Autodesk Inventor part; units mm, degrees
ref_plane "YZ Plane" through (0, 0, 0) normal (1, 0, 0) x (0, 1, 0)
ref_plane "XZ Plane" through (0, 0, 0) normal (0, 1, 0) x (-1, 0, 0)
ref_plane "XY Plane" through (0, 0, 0) normal (0, 0, 1) x (1, 0, 0)
sketch "Sketch1" plane through (0, 0, 0) normal (0, 0, 1) x (1, 0, 0)
  line L0 (0, 0) -> (125, 0)
  line L1 (125, 0) -> (125, 50)
  line L2 (125, 50) -> (0, 50)
  line L3 (0, 50) -> (0, 0)
  dimension "d0" = 125
  dimension "d1" = 50
extrude "Extrusion1" add sketch "Sketch1" along normal blind 10
sketch "Sketch2" plane through (0, 0, 10) normal (0, 0, 1) x (1, 0, 0)
  circle A0 centre (31.25, 25) radius 2.5
  circle A1 centre (93.75, 25) radius 2.5
  line L0 (125, 50) -> (0, 50)
  line L1 (0, 0) -> (125, 0)
  line L2 (125, 0) -> (125, 50)
  line L3 (0, 50) -> (0, 0)
  dimension "d4" = 5
  dimension "d5" = 5
  dimension "d6" = 62.5
  dimension "d7" = 25
  dimension "d8" = 50
  dimension "d9" = 125
  dimension "d10" = 31.25
  dimension "d26" = 25
  dimension "d27" = 31.25
extrude "Extrusion2" cut sketch "Sketch2" against normal blind 5 contours A0 | A1
sketch "Sketch3" plane through (0, 0, 10) normal (0, 0, 1) x (1, 0, 0)
  circle A0 centre (62.5, 40) radius 1
  circle A1 centre (62.5, 10) radius 1
  line L0 (0, 0) -> (125, 0)
  line L1 (125, 50) -> (0, 50)
  line L2 (125, 0) -> (125, 50)
  line L3 (0, 50) -> (0, 0)
  dimension "d13" = 2
  dimension "d14" = 2
  dimension "d16" = 50
  dimension "d17" = 10
  dimension "d20" = 125
  dimension "d23" = 62.5
  dimension "d24" = 62.5
  dimension "d25" = 30
extrude "Extrusion3" cut sketch "Sketch3" against normal blind 10 contours A0 | A1
equation "\"d7\" = 0.5 * d8"
equation "\"d10\" = 0.5 * d9 - 0.5 * d6"
equation "\"d26\" = d7"
equation "\"d17\" = 0.5 * d16 - 0.5 * d25"
equation "\"d23\" = 0.5 * d20"
equation "\"d24\" = d23"
equation "\"d15\" = 0.5 * d16"
properties part number "extremite" material "Wood (Oak)"
Source: CAD feature listing. Evaluate the final solid. Frame: model axes, mm. A direction names the side the tool comes from. Give positions to 0.01 mm unless a question says otherwise; leave off trailing zeros. Order: outer loops, then holes, each group sorted by start corner. A loop starts at its lowest first (then second) coordinate and runs counter-clockwise, first axis right, second up. Notation, with made-up numbers: (4.25, 32.5) -> (43.25, 32.5) arc R13 cw to (43.25, 41.5) -> close; hole circle Ø2 at (83, 36.5). An arc over 180 degrees is marked (long way). Use a Markdown table: item, result.
1) Reachability of faces 4 (the flat face through (31, 25, 5)), 5 (the flat face through (0, 25, 5)) from +Z, -Z, +X, -X, +Y, -Y: full face, straight path, thin tool, end or side. Return the list, or none.
Answer list:
| item | result |
|---|---|
| face 4 | +Z |
| face 5 | +Z, -Z, -X, +Y, -Y |
2) Contact query for flat-ended pins moving along their axis: P1, Ø2.5, axis at x = 93.5, y = 25, coming from the +Z side; P2, Ø6, axis at x = 90.5, y = 15, coming from the -Z side. Output: stop coordinate, or through.
Answer list:
| item | result |
|---|---|
| P1 | z = 5 |
| P2 | z = 0 |
3) Section query B-B, the plane x = 93.75. Return the cut outline in (y, z).
Answer list:
| item | result |
|---|---|
| outline | (0, 0) -> (50, 0) -> (50, 10) -> (27.5, 10) -> (27.5, 5) -> (22.5, 5) -> (22.5, 10) -> (0, 10) -> close |
4) Ray query, line 1 along Y through (x, z) = (62.5, 3.25); line 2 along Y through (x, z) = (93.75, 6.5). Return the intervals inside material, ascending. Write a range as [from, to].
Answer list:
| item | result |
|---|---|
| line 1 | [0, 9], [11, 39], [41, 50] |
| line 2 | [0, 22.5], [27.5, 50] |
5) Mould query, pull axis X, two halves, no side actions, for faces 1 (the flat face through (62, 25, 10)), 2 (the cylindrical face through (91.91, 26.69, 7.54)), 3 (the flat face through (125, 25, 5)). Classes: +X half, -X half, draft (parallel to the pull), parting line (faces both ways), or undercut.
Answer list:
| item | result |
|---|---|
| face 1 | draft |
| face 2 | undercut |
| face 3 | +X half |
6) Section query A-A, the plane y = 25. Return the cut outline in (x, z), then the cut area to 3 significant figures.
Answer list:
| item | result |
|---|---|
| outline | (0, 0) -> (125, 0) -> (125, 10) -> (96.25, 10) -> (96.25, 5) -> (91.25, 5) -> (91.25, 10) -> (33.75, 10) -> (33.75, 5) -> (28.75, 5) -> (28.75, 10) -> (0, 10) -> close |
| area | 1,200 mm² |
